Work out the finished part from the listing and answer in its coordinate system (mm). A direction names the side the tool comes from. Round coordinates to 2 decimals unless told otherwise and drop trailing zeros. Order: outer loops, then holes, each group sorted by start corner. A loop starts at its lowest first (then second) coordinate and runs counter-clockwise, first axis right, second up. Notation, with made-up numbers: (74, -37) - (129, -37) arc R16 ccw to (129, -21) - close; hole circle Ø8 at (42, 12). An arc over 180 degrees is marked (long way). Put each result on its own line as item: value.
```python
from build123d import *

# Parameters (mm, degrees)
SKETCH1_W                      = 168
SKETCH1_H                      = 63
BOSS_EXTRUDE1_DEPTH            = 10
SKETCH2_W                      = 168
SKETCH2_H                      = 63
BOSS_EXTRUDE2_DEPTH            = 2
SKETCH3_W                      = 10
SKETCH3_H                      = 25
CUT_EXTRUDE1_DEPTH             = 111.028405423
SKETCH4_W                      = 10
SKETCH4_H                      = 8
CUT_EXTRUDE2_DEPTH             = 3
CUT_EXTRUDE2_DIRECTION_2_REACH = 114.236
SKETCH6_W                      = 10
SKETCH6_H                      = 1
BOSS_EXTRUDE4_DEPTH            = 31
SKETCH7_R                      = 1.5
BOSS_EXTRUDE5_DEPTH            = 3
SKETCH8_W                      = 10
SKETCH8_H                      = 5
BOSS_EXTRUDE6_DEPTH            = 3
SKETCH9_W                      = 15
SKETCH9_H                      = 10
CUT_EXTRUDE3_DEPTH             = 126.207827231
SKETCH10_W                     = 69
SKETCH10_H                     = 1
BOSS_EXTRUDE7_DEPTH            = 15
SKETCH12_W                     = 3
SKETCH12_H                     = 2
CUT_EXTRUDE5_DEPTH             = 126.207827231
SKETCH13_W                     = 5.3
SKETCH13_H                     = 7
CUT_EXTRUDE6_DEPTH             = 3
BOSS_EXTRUDE8_DEPTH            = 3


with BuildPart() as part:
    # Sketch1 → Boss-Extrude1 (new body)
    with BuildSketch(Plane(origin=(0, 0, 0), x_dir=(1, 0, 0), z_dir=(0, 1, 0))):
        Polygon((0, 34.5), (-87, 34.5), (-87, -34.5), (84, -34.5), (104, -34.5), (104, 34.5), (84, 34.5), align=None)
        Rectangle(SKETCH1_W, SKETCH1_H, mode=Mode.SUBTRACT)
    extrude(amount=BOSS_EXTRUDE1_DEPTH)

    # Sketch2 → Boss-Extrude2 (add)
    with BuildSketch(Plane(origin=(0, 0, 0), x_dir=(1, 0, 0), z_dir=(0, 1, 0))):
        Rectangle(SKETCH2_W, SKETCH2_H)
    extrude(amount=BOSS_EXTRUDE2_DEPTH)

    # Sketch3 → Cut-Extrude1 (cut, through all)
    with BuildSketch(Plane(origin=(0, 10, 0), x_dir=(1, 0, 0), z_dir=(0, 1, 0))):
        with Locations((94, 19)):
            Rectangle(SKETCH3_W, SKETCH3_H)
    cut_extrude1 = extrude(amount=-CUT_EXTRUDE1_DEPTH, mode=Mode.SUBTRACT)

    # Mirror1: Cut-Extrude1 across plane
    add(cut_extrude1.mirror(Plane.XY), mode=Mode.SUBTRACT)

    # Sketch4 → Cut-Extrude2 (cut)
    with BuildSketch(Plane.XY.offset(6.5)):
        with Locations((94, 4)):
            Rectangle(SKETCH4_W, SKETCH4_H)
    cut_extrude2 = extrude(amount=-CUT_EXTRUDE2_DEPTH, mode=Mode.SUBTRACT)

    # Sketch4 → Cut-Extrude2 direction 2 (cut, up to next)
    with BuildSketch(Plane.XY.offset(6.5), mode=Mode.PRIVATE) as cut_extrude2_direction_2_sk1:
        with Locations((94, 4)):
            Rectangle(SKETCH4_W, SKETCH4_H)
    cut_extrude2_direction_2_tool1 = extrude(cut_extrude2_direction_2_sk1.sketch, amount=CUT_EXTRUDE2_DIRECTION_2_REACH, mode=Mode.PRIVATE) & part.part
    cut_extrude2_direction_2 = cut_extrude2_direction_2_tool1.solids().sort_by_distance((94, 4, 6.5))[0]
    add(cut_extrude2_direction_2, mode=Mode.SUBTRACT)

    # Mirror2: Cut-Extrude2, Cut-Extrude2 direction 2 across plane
    add(cut_extrude2.mirror(Plane.XY), mode=Mode.SUBTRACT)
    add(cut_extrude2_direction_2.mirror(Plane.XY), mode=Mode.SUBTRACT)

    # Sketch6 → Boss-Extrude4 (add)
    with BuildSketch(Plane.XY.offset(3.5)):
        with Locations((94, 0.5)):
            Rectangle(SKETCH6_W, SKETCH6_H)
    boss_extrude4 = extrude(amount=BOSS_EXTRUDE4_DEPTH)

    # Mirror5: Boss-Extrude4 across plane
    add(boss_extrude4.mirror(Plane.XY))

    # Sketch7 → Boss-Extrude5 (add)
    with BuildSketch(Plane.XY.offset(3.5)):
        with Locations((94, 4.5)):
            Circle(SKETCH7_R)
    boss_extrude5 = extrude(amount=BOSS_EXTRUDE5_DEPTH)

    # Mirror6: Boss-Extrude5 across plane
    add(boss_extrude5.mirror(Plane.XY))

    # Sketch8 → Boss-Extrude6 (add)
    with BuildSketch(Plane.ZY.offset(87)):
        with Locations((0, 2.5)):
            Rectangle(SKETCH8_W, SKETCH8_H)
    extrude(amount=BOSS_EXTRUDE6_DEPTH)

    # Sketch9 → Cut-Extrude3 (cut, through all)
    with BuildSketch(Plane.XY.offset(34.5)):
        with Locations((96.5, 5)):
            Rectangle(SKETCH9_W, SKETCH9_H)
    extrude(amount=-CUT_EXTRUDE3_DEPTH, mode=Mode.SUBTRACT)

    # Sketch10 → Boss-Extrude7 (add)
    with BuildSketch(Plane(origin=(89, 0, 0), x_dir=(0, 0, -1), z_dir=(1, 0, 0))):
        with Locations((0, 0.5)):
            Rectangle(SKETCH10_W, SKETCH10_H)
    extrude(amount=BOSS_EXTRUDE7_DEPTH)

    # Sketch12 → Cut-Extrude5 (cut, through all)
    with BuildSketch(Plane.XY.offset(34.5)):
        with Locations((87.5, 9)):
            Rectangle(SKETCH12_W, SKETCH12_H)
    extrude(amount=-CUT_EXTRUDE5_DEPTH, mode=Mode.SUBTRACT)

    # Sketch13 → Cut-Extrude6 (cut)
    with BuildSketch(Plane(origin=(89, 0, 0), x_dir=(0, 0, -1), z_dir=(1, 0, 0))):
        with Locations((0, 4.5)):
            Rectangle(SKETCH13_W, SKETCH13_H)
    extrude(amount=-CUT_EXTRUDE6_DEPTH, mode=Mode.SUBTRACT)

    # Sketch15 → Boss-Extrude8 (add)
    with BuildSketch(Plane(origin=(0, 1, 0), x_dir=(1, 0, 0), z_dir=(0, 1, 0))):
        with BuildLine():
            Line((103, 10), (103, -10))
            ThreePointArc((103, -10), (101.5, -11.5), (100, -10))
            Line((100, -10), (100, 10))
            ThreePointArc((100, 10), (101.5, 11.5), (103, 10))
        make_face()
    extrude(amount=BOSS_EXTRUDE8_DEPTH)


solid = part.part
```
1) Given pin 1 Ø1.5 at (x, y) = (-88.5, 2.5) entering from -Z; pin 2 Ø2 at (x, z) = (38.5, -25) entering from +Y; pin 3 Ø2.5 at (y, z) = (3, -3) entering from +X; pin 4 Ø3.5 at (x, z) = (87, 12.5) entering from +Y, each flat-ended and moving along its own axis, determine where each tip first touches the part or whether it passes through.
Findings below:
pin 1: stops at z = -5
pin 2: stops at y = 2
pin 3: stops at x = 103
pin 4: stops at y = 10
2) Straight lines are drawn through the part: L1, parallel to Z at x = -62.5, y = 9.25; L2, parallel to Z at x = 87, y = 7.5; L3, parallel to X at y = 1.5, z = -2.5. For each, find the intervals that lie inside material, in ascending order. Write a range as from..to.
Findings below:
L1: z = -34.5..-31.5, 31.5..34.5
L2: z = -34.5..-2.65, 2.65..34.5
L3: x = -90..86, 100..103
3) A cutting plane is placed at C-C on z = 8. Write down the section's boundary in (x, y).
Findings below:
outline: (-87, 0) - (104, 0) - (104, 1) - (103, 1) - (103, 4) - (100, 4) - (100, 1) - (89, 1) - (89, 8) - (86, 8) - (86, 10) - (84, 10) - (84, 2) - (-84, 2) - (-84, 10) - (-87, 10) - close
4) A cutting plane is placed at B-B on z = 0. Write down the section's boundary in (x, y), then the cut area to 3 significant figures.
Findings below:
outline: (-90, 0) - (104, 0) - (104, 1) - (103, 1) - (103, 4) - (100, 4) - (100, 1) - (86, 1) - (86, 10) - (84, 10) - (84, 2) - (-84, 2) - (-84, 10) - (-87, 10) - (-87, 5) - (-90, 5) - close
area: 428 mm2
5) A cutting plane is placed at A-A on x = 14. Write down the section's boundary in (y, z), then the cut area to 3 significant figures.
Findings below:
outline: (0, -34.5) - (10, -34.5) - (10, -31.5) - (2, -31.5) - (2, 31.5) - (10, 31.5) - (10, 34.5) - (0, 34.5) - close
area: 186 mm2
6) A cutting plane is placed at D-D on z = -27.5. Write down the section's boundary in (x, y).
Findings below:
outline: (-87, 0) - (104, 0) - (104, 1) - (89, 1) - (89, 8) - (86, 8) - (86, 10) - (84, 10) - (84, 2) - (-84, 2) - (-84, 10) - (-87, 10) - close
7) For faces 1 (the flat face through (6, 0, 0)), 2 (the flat face through (-84, 6, 0)), determine the directions among +Z, -Z, +X, -X, +Y, -Y from which every point of the face is accessible in a straight line to the end or side of a thin tool.
Findings below:
face 1: +Z, -Z, +X, -X, -Y
face 2: +Y
8) For a pull along X with two mould halves and no side action, classify faces 3 (the flat face through (-90, 3, 0)), 4 (the flat face through (89, 4, -18)), 5 (the flat face through (7, 5, -34.5)) as pulls with the +X half, pulls with the -X half, needs draft (parallel to the pull), parting line crosses it, or undercut.
Findings below:
face 3: pulls with the -X half
face 4: undercut
face 5: needs draft
